Build history of the part. All positions in model axes, mm. Face numbers are marked on the shaded views. A direction names the side the tool comes from. Coordinates: 2 decimals unless noted, no trailing zeros. Loops run counter-clockwise (first coordinate to the right, second up) from the corner with the lowest first, then second, coordinate; pieces in that order, holes last. Notation, with made-up numbers: (-13.75, -1) - (-2.75, -1) arc R8 cw to (-2.75, 10) - close; hole circle Ø3 at (89, -17). An arc over 180 degrees is marked (long way). One line per item, written item: value.
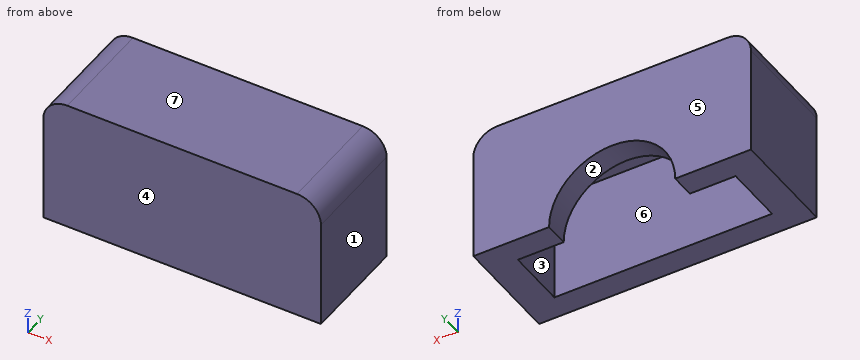
Autodesk Inventor part; units mm, degrees
ref_plane "YZ Plane" through (0, 0, 0) normal (1, 0, 0) x (0, 1, 0)
ref_plane "XZ Plane" through (0, 0, 0) normal (0, 1, 0) x (-1, 0, 0)
ref_plane "XY Plane" through (0, 0, 0) normal (0, 0, 1) x (1, 0, 0)
ref_plane "Arbeitsebene1" through (-12.85, 3.6, -4.5) normal (0, -1, 0) x (0, 0, 1)
sketch "Skizze1" plane through (-12.85, 3.6, -4.5) normal (0, -1, 0) x (0, 0, 1)
  circle A0 centre (0, 0) radius 4.3 construction
  line L0 (0.4805, 5.7801) -> (0.4805, 4.5246)
  line L1 (0.4805, -4.5246) -> (0.4805, -5.7801)
  line L2 (0, -5.8) -> (5.55, -5.8)
  line L3 (5.55, -5.8) -> (5.55, 5.8)
  line L4 (5.55, 5.8) -> (0, 5.8)
  line L5 (0, 5.8) -> (0, -5.8)
  line L6 (0, -4.55) -> (4.55, -4.55)
  line L7 (4.55, -4.55) -> (4.55, 4.55)
  line L8 (4.55, 4.55) -> (0, 4.55)
  line L9 (0, 4.55) -> (0, -4.55)
  point P0 (4.5, -12.85)
  point P1 (0, 4.55)
  dimension "d2" = 0
  dimension "d27" = 0
  dimension "d28" = 1
extrude "Extrusion1" add sketch "Skizze1" along normal blind 2.5 contours L5 L6 L7 L8 L4 L3 L2
sketch "Skizze2" plane through (-12.85, 1.1, -4.5) normal (0, -1, 0) x (1, 0, 0)
  line L0 (-5.7801, 0.4805) -> (5.7801, 0.4805)
  line L1 (-5.8, 0) -> (-4.55, 0)
  line L2 (-4.55, 0) -> (-4.55, 4.55)
  line L3 (-4.55, 4.55) -> (4.55, 4.55)
  line L4 (4.55, 4.55) -> (4.55, 0)
  line L5 (4.55, 0) -> (5.8, 0)
  line L6 (5.8, 0) -> (5.8, 5.55)
  line L7 (5.8, 5.55) -> (-5.8, 5.55)
  line L8 (-5.8, 5.55) -> (-5.8, 0)
  line L9 (-4.55, 0) -> (4.55, 0)
  point P0 (12.85, 4.5)
extrude "Extrusion2" add sketch "Skizze2" along normal blind 1
sketch "Skizze7" plane through (-12.85, 3.6, -4.5) normal (0, 1, 0) x (1, 0, 0)
  line L0 (-5.8, 0) -> (-4.55, 0)
  line L1 (-5.8, -5.55) -> (-5.8, 0)
  line L2 (5.8, -5.55) -> (-5.8, -5.55)
  line L3 (5.8, 0) -> (5.8, -5.55)
  line L4 (4.55, 0) -> (5.8, 0)
  line L5 (4.55, -4.55) -> (4.55, 0)
  line L6 (-4.55, -4.55) -> (4.55, -4.55)
  line L7 (-4.55, 0) -> (-4.55, -4.55)
  line L8 (4.55, 0) -> (-4.55, 0)
  line L9 (-4.55, -4.55) -> (4.55, -4.55)
  circle A0 centre (0, 0) radius 2.6359
  point P0 (12.85, -4.5)
  point P1 (2.6359, 0)
  point P2 (-2.6359, 0)
extrude "Extrusion6" add sketch "Skizze7" along normal blind 1 contours L0 L7 L6 L5 L4 L3 L2 L1 | L8 A0 L5 L6 L7
fillet "Rundung2" radius 1 2 edges at (-18.65, 2.35, 1.05) (-7.05, 2.35, 1.05)
properties part number "20_Cube_Insert_Syringepump_Micro_syringeclamp_v3"
Item 1: Drop a flat-ended pin along its axis: P1, Ø1.2, axis at x = -14.5, y = 2.5, coming from the -Z side. Give the stop position or say it passes through.
Check result:
P1: stops at z = 0.05
Item 2: Pull direction Y, two halves, no side cores. Call the marked faces 4, 5, 6 and 7: released by +Y, released by -Y, zero draft, split by the parting line, or undercut.
Check result:
face 4: released by -Y
face 5: released by +Y
face 6: undercut
face 7: zero draft
Item 3: Cut at A-A, the plane z = -1.6. Write the cut outline in (x, y).
Check result:
outline: (-18.65, 0.1) - (-7.05, 0.1) - (-7.05, 4.6) - (-18.65, 4.6) - close; hole (-17.4, 1.1) - (-8.3, 1.1) - (-8.3, 3.6) - (-17.4, 3.6) - close
Item 4: Cut at C-C, the plane y = 2.6. Write the cut outline in (x, z).
Check result:
outline: (-18.65, -4.5) - (-17.4, -4.5) - (-17.4, 0.05) - (-8.3, 0.05) - (-8.3, -4.5) - (-7.05, -4.5) - (-7.05, 0.05) arc R1 ccw to (-8.05, 1.05) - (-17.65, 1.05) arc R1 ccw to (-18.65, 0.05) - close
Item 5: Probe probe 1 along Y at (x, z) = (-15.75, -2.15); probe 2 along X at (y, z) = (2.45, -0.45); probe 3 along Y at (x, z) = (-11.5, -3.6). List the from-to ranges inside material, lowest first. Write a range as from..to.
Check result:
probe 1: y = 0.1..1.1, 3.6..4.6
probe 2: x = -18.65..-17.4, -8.3..-7.05
probe 3: y = 0.1..1.1
Item 6: Cut at B-B, the plane x = -12.85. Write the cut outline in (y, z), then the cut area to 3 significant figures.
Check result:
outline: (0.1, -4.5) - (1.1, -4.5) - (1.1, 0.05) - (3.6, 0.05) - (3.6, -1.86) - (4.6, -1.86) - (4.6, 1.05) - (0.1, 1.05) - close
area: 11.0 mm^2
Item 7: Tool access for the marked faces 1, 2 and 3: list every direction of +Z, -Z, +X, -X, +Y, -Y with a clear straight run to the whole face (end or side of a thin tool).
Check result:
face 1: +Z, -Z, +X, +Y, -Y
face 2: -Z, +Y
face 3: -Z
